Geometry check sheet. Reference: the model listing, model coordinates, mm. A direction names the side the tool comes from. Coordinates: 2 decimals unless noted, no trailing zeros. Write each loop counter-clockwise with the first axis right and the second up, starting at its lowest first coordinate (ties: lowest second). Pieces come first, ordered by that corner, then holes. Notation, with made-up numbers: (34.5, 57) -> (43.5, 57) arc R23 cw to (43.5, 87) -> close; hole circle Ø2 at (48.25, -18.5). An arc over 180 degrees is marked (long way). One line per question, with ' | ' between items.
from build123d import *

# Parameters (mm, degrees)
SKETCH1_R           = 40
BOSS_EXTRUDE1_DEPTH = 12
SKETCH2_R           = 25
CUT_EXTRUDE1_DEPTH  = 58.827329179
SKETCH3_R           = 4
CUT_EXTRUDE2_DEPTH  = 58.827329179
CUT_EXTRUDE3_START  = -4
SKETCH4_R           = 27
SKETCH4_R_2         = 25
CUT_EXTRUDE3_DEPTH  = 4


with BuildPart() as part:
    # Sketch1 → Boss-Extrude1 (new body)
    with BuildSketch(Plane.XY):
        Circle(SKETCH1_R)
    extrude(amount=BOSS_EXTRUDE1_DEPTH)

    # Sketch2 → Cut-Extrude1 (cut, through all)
    with BuildSketch(Plane(origin=(0, 0, 0), x_dir=(-1, 0, 0), z_dir=(0, 0, -1))):
        Circle(SKETCH2_R)
    extrude(amount=-CUT_EXTRUDE1_DEPTH, mode=Mode.SUBTRACT)

    # Sketch3 → Cut-Extrude2 (cut, through all)
    with BuildSketch(Plane.XY.offset(12)):
        with Locations((-33, 0)):
            Circle(SKETCH3_R)
        with Locations((0, 33)):
            Circle(SKETCH3_R)
        with Locations((33, 0)):
            Circle(SKETCH3_R)
        with Locations((0, -33)):
            Circle(SKETCH3_R)
    extrude(amount=-CUT_EXTRUDE2_DEPTH, mode=Mode.SUBTRACT)

    # Sketch4 → Cut-Extrude3 (cut)
    with BuildSketch(Plane.XY.offset(12).offset(CUT_EXTRUDE3_START)):
        Circle(SKETCH4_R)
        with Locations(Location((0, 0, 0), (0, 0, 180))):
            Circle(SKETCH4_R_2, mode=Mode.SUBTRACT)
    extrude(amount=CUT_EXTRUDE3_DEPTH, mode=Mode.SUBTRACT)


solid = part.part
1. Cross-section at A-A on y = 0. Record the boundary of the cut face in (x, z).
Worked answers:
outline: (-40, 0) -> (-37, 0) -> (-37, 12) -> (-40, 12) -> close; (-29, 0) -> (-25, 0) -> (-25, 8) -> (-27, 8) -> (-27, 12) -> (-29, 12) -> close; (25, 0) -> (29, 0) -> (29, 12) -> (27, 12) -> (27, 8) -> (25, 8) -> close; (37, 0) -> (40, 0) -> (40, 12) -> (37, 12) -> close
2. Tool access check on faces 1 (the face through (-36.2, -2.4, 6.1)), 2 (the face through (-5.85, -26.36, 9.97)). Record the directions out of +Z, -Z, +X, -X, +Y, -Y that give a thin tool (end or side, any length) a straight path to the whole face; none if there is none.
Worked answers:
face 1: +Z, -Z | face 2: +Z
3. Mould release check, pull along X, two halves, no side actions. Record for faces 3 (the face through (24, -8, 8)), 4 (the face through (8, -26, 12)), 5 (the face through (-8.67, -39.05, 5.92)): released by +X, released by -X, zero draft, split by the parting line, or undercut.
Worked answers:
face 3: undercut | face 4: zero draft | face 5: split by the parting line
4. Cross-section at C-C on x = -33. Record the boundary of the cut face in (y, z).
Worked answers:
outline: (-22.61, 0) -> (-4, 0) -> (-4, 12) -> (-22.61, 12) -> close; (4, 0) -> (22.61, 0) -> (22.61, 12) -> (4, 12) -> close
5. Cross-section at D-D on y = -22. Record the boundary of the cut face in (x, z), and give its area (3 significant figures).
Worked answers:
outline: (-33.41, 0) -> (-11.87, 0) -> (-11.87, 8) -> (-15.65, 8) -> (-15.65, 12) -> (-33.41, 12) -> close; (11.87, 0) -> (33.41, 0) -> (33.41, 12) -> (15.65, 12) -> (15.65, 8) -> (11.87, 8) -> close | area: 487 mm²
6. Material ranges on line 1 (Y direction, x = 0, z = 10.7); line 2 (Y direction, x = 0, z = 4.5); line 3 (X direction, y = -5.5, z = 11.25), recorded low to high. Write a range as from..to.
Worked answers:
line 1: -40..-37, -29..-27, 27..29, 37..40 | line 2: -40..-37, -29..-25, 25..29, 37..40 | line 3: -39.62..-26.43, 26.43..39.62
7. Go/stop test with flat-tipped pins: P1, Ø6.5, axis at x = -33, y = 0, coming from the +Z side; P2, Ø5, axis at y = -29.5, z = 3, coming from the -X side; P3, Ø4, axis at y = 6, z = 1.5, coming from the +X side; P4, Ø4, axis at x = -24.5, z = 9.5, coming from the +Y side. Record where each tip stops, or that it passes through.
Worked answers:
P1: through | P2: x = -29.51 | P3: x = 39.8 | P4: y = 33.07
